from build123d import *

# Parameters (mm, degrees)
SKETCH_1_W             = 60
SKETCH_1_H             = 310
EXTRUDE_1_DEPTH        = 6
SKETCH_2_R             = 3.3
CUT_EXTRUDE_1_DEPTH    = 158.990506044
CHAMFER_2_SIZE         = 5
CHAMFER_1_SIZE         = 1
HOLE_WIZARD_M6_1_D     = 5
HOLE_WIZARD_M6_1_DEPTH = 19.75
HOLE_WIZARD_M6_1_TIP   = 1.502151548


with BuildPart() as part:
    # 草图1 → 凸台-拉伸1 (new body)
    with BuildSketch(Plane.XY):
        Rectangle(SKETCH_1_W, SKETCH_1_H)
    extrude(amount=EXTRUDE_1_DEPTH)

    # 草图2 → 切除-拉伸1 (cut, through all)
    with BuildSketch(Plane.XY.offset(6)):
        with Locations((-20, 135)):
            Circle(SKETCH_2_R)
        with Locations((20, 135)):
            Circle(SKETCH_2_R)
        with Locations((-20, -135)):
            Circle(SKETCH_2_R)
        with Locations((20, -135)):
            Circle(SKETCH_2_R)
    extrude(amount=-CUT_EXTRUDE_1_DEPTH, mode=Mode.SUBTRACT)

    # 倒角2
    chamfer_2_edges = [part.edges().sort_by_distance(p)[0] for p in [
        (30, -155, 3),
        (-30, -155, 3),
        (-30, 155, 3),
        (30, 155, 3),
    ]]
    chamfer(chamfer_2_edges, length=CHAMFER_2_SIZE)

    # 倒角1
    chamfer_1_edges = [part.edges().sort_by_distance(p)[0] for p in [
        (0, -155, 0),
        (0, -155, 6),
        (30, 0, 0),
        (-30, 0, 0),
        (0, 155, 0),
        (27.5, 152.5, 0),
        (-27.5, 152.5, 0),
        (27.5, -152.5, 0),
        (-27.5, -152.5, 0),
        (-30, 0, 6),
        (30, 0, 6),
        (0, 155, 6),
        (27.5, 152.5, 6),
        (-27.5, 152.5, 6),
        (27.5, -152.5, 6),
        (-27.5, -152.5, 6),
    ]]
    chamfer(chamfer_1_edges, length=CHAMFER_1_SIZE)

    # M6 螺纹孔1
    with Locations(Plane(origin=(0, 0, 0), x_dir=(-1, 0, 0), z_dir=(0, 0, -1))):
        with Locations((-20, 89.999999889), (20, 89.999999889), (20, -90.000000111), (-20, -90.000000111)):
            Hole(HOLE_WIZARD_M6_1_D / 2, depth=HOLE_WIZARD_M6_1_DEPTH)
            with Locations((0, 0, -(HOLE_WIZARD_M6_1_DEPTH + HOLE_WIZARD_M6_1_TIP / 2))):  # 118° drill point
                Cone(0, HOLE_WIZARD_M6_1_D / 2, HOLE_WIZARD_M6_1_TIP, mode=Mode.SUBTRACT)


solid = part.part
Build history of the part. All positions in model axes, mm. Give positions to 0.01 mm unless a question says otherwise; leave off trailing zeros. Order: outer loops, then holes, each group sorted by start corner. A loop starts at its lowest first (then second) coordinate and runs counter-clockwise, first axis right, second up. Notation, with made-up numbers: M 66.5,21 L 92.5,21 A18 cw 92.5,49 Z; hole C 76.5,66 d2. An arc over 180 degrees is marked long. Use one line per item in the form item = value.
1) Probe probe 1 along Y at (x, z) = (-20, 2.8); probe 2 along X at (y, z) = (90, 4.8); probe 3 along Y at (x, z) = (19, 5.75). List the from-to ranges inside material, lowest first.
Calculated:
probe_1 = -155 to -138.3, -131.7 to -92.5, -87.5 to 87.5, 92.5 to 131.7, 138.3 to 155
probe_2 = -30 to -22.5, -17.5 to 17.5, 22.5 to 30
probe_3 = -154.25 to -138.14, -131.86 to -92.29, -87.71 to 87.71, 92.29 to 131.86, 138.14 to 154.25
2) Drop a flat-ended pin along its axis: pin 1 (3 mm diameter, centred on x = -20, y = 90, fed in from +Z). Give the stop position or say it passes through.
Calculated:
pin_1 = through
3) Saw through at A-A (y = 135). Give the cut face in (x, z).
Calculated:
outline = M -30,1 L -29,0 L -23.3,0 L -23.3,6 L -29,6 L -30,5 Z; M -16.7,0 L 16.7,0 L 16.7,6 L -16.7,6 Z; M 23.3,0 L 29,0 L 30,1 L 30,5 L 29,6 L 23.3,6 Z
4) Two-plate mould, pull along X, no slides. Class faces 1 (the face through (0, 2, 0)), 2 (the face through (19.46, -92.44, 3.04)), 3 (the face through (27.12, 152.19, 0.51)), 4 (the face through (19.28, 131.78, 3.04)): released by +X, released by -X, zero draft, split by the parting line, or undercut.
Calculated:
face_1 = zero draft
face_2 = undercut
face_3 = released by +X
face_4 = undercut
